from build123d import *

# Parameters (mm, degrees)
EXTRUDE_1_DEPTH = 8
SKETCH_2_R      = 5
EXTRUDE_2_DEPTH = 220
CHAMFER_1_SIZE  = 2
CHAMFER_1_SIZE2 = 1.154700538


with BuildPart() as part:
    # Эскиз1 → Бобышка-Вытянуть1 (new body)
    with BuildSketch(Plane(origin=(0, 0, 0), x_dir=(1, 0, 0), z_dir=(0, 1, 0))):
        Polygon((8.5, -4.907477288), (8.5, 4.907477288), (0, 9.814954576), (-8.5, 4.907477288), (-8.5, -4.907477288), (0, -9.814954576), align=None)
    extrude(amount=EXTRUDE_1_DEPTH)

    # Эскиз2 → Бобышка-Вытянуть2 (add)
    with BuildSketch(Plane(origin=(0, 8, 0), x_dir=(1, 0, 0), z_dir=(0, 1, 0))):
        Circle(SKETCH_2_R)
    extrude(amount=EXTRUDE_2_DEPTH)

    # Фаска1
    chamfer_1_edges = [part.edges().sort_by_distance(p)[0] for p in [
        (-4.25, 0, 7.361215932),
        (-8.5, 0, 0),
        (-4.25, 0, -7.361215932),
        (4.25, 0, -7.361215932),
        (8.5, 0, 0),
        (4.25, 0, 7.361215932),
    ]]
    chamfer_1_side = [part.faces().sort_by_distance(p)[0] for p in [
        (0, 0, 0),
    ]]
    chamfer(chamfer_1_edges, length=CHAMFER_1_SIZE, length2=CHAMFER_1_SIZE2, reference=chamfer_1_side[0])


solid = part.part
Build history of the part. All positions in model axes, mm. A direction names the side the tool comes from. Give positions to 0.01 mm unless a question says otherwise; leave off trailing zeros. Order: outer loops, then holes, each group sorted by start corner. A loop starts at its lowest first (then second) coordinate and runs counter-clockwise, first axis right, second up. Notation, with made-up numbers: M 61.5,54 L 90.5,54 A17 ccw 90.5,68 Z; hole C -35,-7 d5. An arc over 180 degrees is marked long. Put each result on its own line as item: value.
Item 1: Cut at C-C on y = 107.5. Write the cut outline in (x, z).
Results are:
outline: C 0,0 d10
Item 2: Wall check: probe 1 along Y at (x, z) = (5.25, 3.25); probe 2 along X at (y, z) = (116.5, -0.25); probe 3 along Z at (x, y) = (-1, 47). Give the ranges that are in metal, low to high.
Results are:
probe 1: 0 to 8
probe 2: -4.99 to 4.99
probe 3: -4.9 to 4.9
Item 3: Drop flat-ended pins along their axis: pin 1 Ø8 at (x, y) = (0.5, 115.5) entering from +Z; pin 2 Ø6 at (x, y) = (-0.5, 200) entering from -Z; pin 3 Ø4 at (x, y) = (4.5, 139.5) entering from +Z. Give the stop position or say it passes through.
Results are:
pin 1: z = 5
pin 2: z = -5
pin 3: z = 4.33
Item 4: Which spindle directions (+Z, -Z, +X, -X, +Y, -Y) get a long thin tool onto all of the face, cutting with end or side? Do faces 1 (the face through (4, 8, 4)), 2 (the face through (-3.698, 0.585, -6.542)). Say none if no direction does.
Results are:
face 1: +Y
face 2: -Z, -X, -Y
Item 5: Cut at A-A on z = 0. Write the cut outline in (x, y).
Results are:
outline: M -8.5,1.15 L -6.5,0 L 6.5,0 L 8.5,1.15 L 8.5,8 L 5,8 L 5,228 L -5,228 L -5,8 L -8.5,8 Z
Item 6: Cut at B-B on x = 2.5. Write the cut outline in (y, z).
Results are:
outline: M 0,-6.06 L 1.15,-8.37 L 8,-8.37 L 8,-4.33 L 228,-4.33 L 228,4.33 L 8,4.33 L 8,8.37 L 1.15,8.37 L 0,6.06 Z
